Part model, mm, in its own coordinate system. Coordinates: 2 decimals unless noted, no trailing zeros. Loops run counter-clockwise (first coordinate to the right, second up) from the corner with the lowest first, then second, coordinate; pieces in that order, holes last. Notation, with made-up numbers: (-33, 79) -> (17, 79) arc R17 ccw to (17, 87) -> close; hole circle Ø6 at (-23, 82). An arc over 180 degrees is marked (long way). Use one line per item in the form item = value. Start each with the question number.
(1) Drill centre lines: L1, parallel to X at y = 2.05, z = 0; L2, parallel to X at y = 1.75, z = -1.25; L3, parallel to Z at x = 48.5, y = 2.7. Where is each one in solid material? Low to high. Write a range as [from, to].
(2) Band-saw the part on A-A on x = 0. Give the cut face in (y, z), then the cut area to 3 significant figures.
(3) Band-saw the part on B-B on z = 0. Give the cut face in (x, y), then the cut area to 3 significant figures.
(4) Band-saw the part on D-D on z = -4.25. Give the cut face in (x, y), then the cut area to 3 significant figures.
(5) Mould opens along X. For faces 1 (the flat face through (1, 3, 3)), 2 (the cylindrical face through (-51.774, 1.521, 0.923)), 3 (the cylindrical face through (57.5, 1.48, -0.16)), 4 (the cylindrical face through (-57.5, 1.48, 0.16)) say: +X half, -X half, draft (parallel to the pull), parting line (faces both ways), or undercut.
(6) Band-saw the part on C-C on y = 2.1. Give the cut face in (x, z).
(7) Pin check, flat tip, straight feed: P1, Ø2.5, axis at x = 0, z = 0, coming from the -Y side. Stop position of the tip, or through.
```python
from build123d import *

# Parameters (mm, degrees)
BOSS_EXTRUDE1_DEPTH = 3
SKETCH4_R           = 2
CUT_EXTRUDE1_DEPTH  = 10
SKETCH5_R           = 2
CUT_EXTRUDE2_DEPTH  = 10


with BuildPart() as part:
    # Sketch1 → Boss-Extrude1 (new body)
    with BuildSketch(Plane(origin=(0, 0, 0), x_dir=(1, 0, 0), z_dir=(0, 1, 0))):
        with BuildLine():
            Line((50, -7.5), (-50, -7.5))
            ThreePointArc((-50, -7.5), (-57.5, 0), (-50, 7.5))
            Line((-50, 7.5), (50, 7.5))
            ThreePointArc((50, 7.5), (57.5, 0), (50, -7.5))
        make_face()
    extrude(amount=BOSS_EXTRUDE1_DEPTH)

    # Sketch4 → Cut-Extrude1 (cut)
    with BuildSketch(Plane(origin=(0, 3, 0), x_dir=(1, 0, 0), z_dir=(0, 1, 0))):
        with Locations(Location((-50, 0, 0), (0, 0, 270))):
            Circle(SKETCH4_R)
        with Locations(Location((50, 0, 0), (0, 0, 270))):
            Circle(SKETCH4_R)
    extrude(amount=-CUT_EXTRUDE1_DEPTH, mode=Mode.SUBTRACT)

    # Sketch5 → Cut-Extrude2 (cut)
    with BuildSketch(Plane(origin=(0, 3, 0), x_dir=(1, 0, 0), z_dir=(0, 1, 0))):
        with Locations(Location((0, 0, 0), (0, 0, 270))):
            Circle(SKETCH5_R)
    extrude(amount=-CUT_EXTRUDE2_DEPTH, mode=Mode.SUBTRACT)


solid = part.part
```
A:
q1.L1 = [-57.5, -52], [-48, -2], [2, 48], [52, 57.5]
q1.L2 = [-57.4, -51.56], [-48.44, -1.56], [1.56, 48.44], [51.56, 57.4]
q1.L3 = [-7.5, -1.32], [1.32, 7.5]
q2.outline = (0, -7.5) -> (3, -7.5) -> (3, -2) -> (0, -2) -> close; (0, 2) -> (3, 2) -> (3, 7.5) -> (0, 7.5) -> close
q2.area = 33.0 mm²
q3.outline = (-57.5, 0) -> (-52, 0) -> (-52, 3) -> (-57.5, 3) -> close; (-48, 0) -> (-2, 0) -> (-2, 3) -> (-48, 3) -> close; (2, 0) -> (48, 0) -> (48, 3) -> (2, 3) -> close; (52, 0) -> (57.5, 0) -> (57.5, 3) -> (52, 3) -> close
q3.area = 309 mm²
q4.outline = (-56.18, 0) -> (56.18, 0) -> (56.18, 3) -> (-56.18, 3) -> close
q4.area = 337 mm²
q5.face_1 = draft
q5.face_2 = undercut
q5.face_3 = +X half
q5.face_4 = -X half
q6.outline = (-50, -7.5) -> (50, -7.5) arc R7.5 ccw to (50, 7.5) -> (-50, 7.5) arc R7.5 ccw to start; hole circle Ø4 at (-50, 0); hole circle Ø4 at (0, 0); hole circle Ø4 at (50, 0)
q7.P1 = through
